```python
from build123d import *

# Parameters (mm, degrees)
F0_W      = 87.3125
F0_H      = 57.15
F1_DEPTH  = 31.75
F3_DEPTH  = 12.7
F4_W      = 8.73125
F4_H      = 6.35
F5_DEPTH  = 66.294
F6_R      = 1.58749
F7_R      = 3.175
F8_R      = 6.35
F9_DEPTH  = 108.204
F10_R     = 4.7625
F11_DEPTH = 12.7


# Not quite as in the source:
# - a fillet or chamfer is up to 0.001 mm smaller than in the source, because OpenCascade refuses the exact size


with BuildPart() as f1:
    # F0 (on Front) → F1 (new body)
    with BuildSketch(Plane.XZ):
        with Locations((43.65625, -28.575)):
            Rectangle(F0_W, F0_H)
    extrude(amount=F1_DEPTH)

    # F2 (on face) → F3 (cut)
    with BuildSketch(Plane.XZ.offset(31.75)):
        Polygon((50.8, -36.5125), (50.8, -57.15), (81.9624807795, -57.15), (59.048891971, -17.4625), (59.048891971, -10.31875), (65.0064250612, 0), (29.7194982962, 0), align=None)
    extrude(amount=-F3_DEPTH, mode=Mode.SUBTRACT)

    # F4 (on face) → F5 (cut)
    with BuildSketch(Plane.XY):
        Polygon((87.3125, 0), (24.60625, 0), (24.60625, -6.35), (33.3375, -6.35), (33.3375, -7.9375), (87.3125, -7.9375), align=None)
        with Locations((4.365625, -3.175)):
            Rectangle(F4_W, F4_H)
    extrude(amount=-F5_DEPTH, mode=Mode.SUBTRACT)

    # F6 (radius 1.5875 in the source; OpenCascade refuses exactly that, so slightly less here)
    f6_edges = [f1.edges().sort_by_distance(p)[0] for p in [
        (33.3375, -7.9375, -28.575),
    ]]
    fillet(f6_edges, radius=F6_R)

    # F7
    f7_edges = [f1.edges().sort_by_distance(p)[0] for p in [
        (87.3125, -19.84375, 0),
        (0, -19.05, 0),
        (87.3125, -19.84375, -57.15),
        (0, -19.05, -57.15),
    ]]
    fillet(f7_edges, radius=F7_R)

    # F8 (on face) → F9 (cut)
    with BuildSketch(Plane.XZ.offset(31.75)):
        with Locations((15.875, -12.7)):
            Circle(F8_R)
        with Locations((15.875, -44.45)):
            Circle(F8_R)
    extrude(amount=-F9_DEPTH, mode=Mode.SUBTRACT)

    # F10 (on face) → F11 (cut)
    with BuildSketch(Plane.YZ.offset(87.3125)):
        with Locations((-19.84375, -28.575)):
            Circle(F10_R)
    extrude(amount=-F11_DEPTH, mode=Mode.SUBTRACT)


solid = f1.part
```
Read the model definition and answer for the solid it produces. Units are mm, in the model's axes. A direction names the side the tool comes from. Round coordinates to 2 decimals unless told otherwise and drop trailing zeros. Write each loop counter-clockwise with the first axis right and the second up, starting at its lowest first coordinate (ties: lowest second). Pieces come first, ordered by that corner, then holes. Notation, with made-up numbers: (-35, 83) - (-26, 83) arc R26 ccw to (-26, 104) - close; hole circle Ø1 at (83.5, -31.75). An arc over 180 degrees is marked (long way). One line per item, written item: value.
Q1. Find section A-A (y = -26.5). Count the separate pieces of the cut face and the enclosed holes in it, and give its area (3 significant figures).
The answers:
separate pieces: 2
enclosed holes: 2
area: 3,390 mm2
Q2. Each of these flat-tipped pins is pushed along its axis until it touches: P1, Ø1.5, axis at x = 45, z = -16.5, coming from the -Y side; P2, Ø1, axis at x = 36, z = -32.5, coming from the +Y side; P3, Ø1.9, axis at y = -3.5, z = -18.5, coming from the -X side. Where does it stop, or does it pass through?
The answers:
P1: stops at y = -19.05
P2: stops at y = -7.94
P3: stops at x = 8.73
Q3. Straight lines are drawn through the part: line 1 (Z direction, x = 21.5, y = -28); line 2 (Z direction, x = 20, y = -9); line 3 (Y direction, x = 35.5, z = -15). For each, find the intervals that lie inside material, in ascending order. Write a range as from..to.
The answers:
line 1: z = -57.15..-47.4, -41.5..-15.65, -9.75..0
line 2: z = -57.15..-49.28, -39.62..-17.53, -7.87..0
line 3: y = -31.75..-7.94
Q4. Find section C-C (y = -3). Determine the outline of the cut face in (x, z) (3 decimals), and give its area (3 significant figures).
The answers:
outline: (8.731, -57.15) - (24.606, -57.15) - (24.606, 0) - (8.731, 0) - close; hole circle Ø12.7 at (15.875, -44.45); hole circle Ø12.7 at (15.875, -12.7)
area: 654 mm2
Q5. Find section D-D (x = 64). Determine the outline of the cut face in (y, z), and give its area (3 significant figures).
The answers:
outline: (-31.75, -26.04) - (-19.05, -26.04) - (-19.05, -57.15) - (-7.94, -57.15) - (-7.94, 0) - (-19.05, 0) - (-19.05, -1.74) - (-31.75, -1.74) - close
area: 944 mm2
Q6. Which of the six approach directions +Z, -Z, +X, -X, +Y, -Y give full straight-line access (tool end or side, diameter ignored) to faces 4 (the flat face through (40.11, -25.49, -18)), 5 (the flat face through (70.666, -25.489, -37.584)), 6 (the flat face through (8.731, -3, -28)), 7 (the flat face through (74.612, -20, -29))?
The answers:
face 4: +Z, -Y
face 5: -Z, -Y
face 6: +Z, -Z, -X, +Y
face 7: +X
Q7. For a pull along X with two mould halves and no side action, classify faces 1 (the cylindrical face through (0.91, -19.23, -56.2)), 2 (the flat face through (59.049, -25, -14)), 3 (the flat face through (76, -31.75, -22)) as pulls with the +X half, pulls with the -X half, needs draft (parallel to the pull), parting line crosses it, or undercut.
The answers:
face 1: pulls with the -X half
face 2: undercut
face 3: needs draft
